```python
from build123d import *

# Parameters (mm, degrees)
F0_W     = 47.9163888
F0_H     = 16.881729
F1_DEPTH = 12.7
F2_R     = 8.382
F3_SIZE  = 8.382


# Not quite as in the source:
# - a feature names something its author has since deleted; it is built from what else it names


with BuildPart() as f1:
    # F0 (on Front) → F1 (new body, symmetric)
    with BuildSketch(Plane.XZ):
        Rectangle(F0_W, F0_H)
    extrude(amount=F1_DEPTH, both=True)

    # F2
    f2_edges = [f1.edges().sort_by_distance(p)[0] for p in [
        (0, -12.7, 8.440864),
        (0, -12.7, -8.440865),
        (-23.958194, -12.7, 0),
        (23.958194, -12.7, 0),
    ]]
    fillet(f2_edges, radius=F2_R)

    # F3
    f3_edges = [f1.edges().sort_by_distance(p)[0] for p in [
        (0, 12.7, 8.440864),
        (23.958194, 12.7, 0),
        (0, 12.7, -8.440865),
        (-23.958194, 12.7, 0),
    ]]
    chamfer(f3_edges, length=F3_SIZE)


solid = f1.part
```
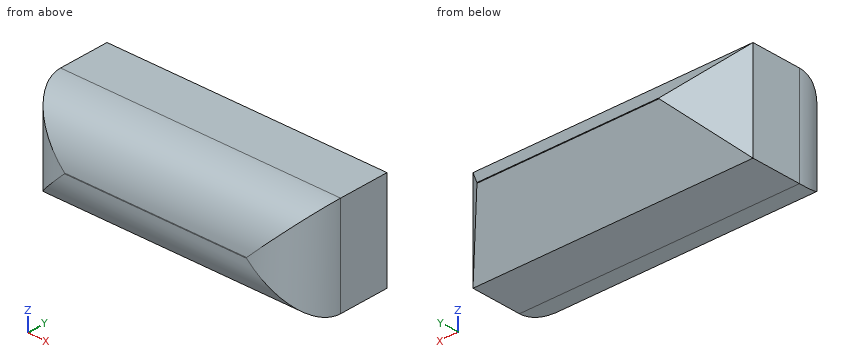
The listing builds one solid part. Answer for the finished solid, in the listing's coordinates (mm). Give positions to 0.01 mm unless a question says otherwise; leave off trailing zeros. Loops run counter-clockwise (first coordinate to the right, second up) from the corner with the lowest first, then second, coordinate; pieces in that order, holes last. Notation, with made-up numbers: (67.5, -16.5) - (108.5, -16.5) arc R15 ccw to (108.5, 10.5) - close; hole circle Ø1 at (-32, 31.25). An arc over 180 degrees is marked (long way). Return JSON: item names as keys, results as strings. Group by question number.
1. Find section B-B (z = 2.75). Write down the section's boundary in (x, y), then the cut area to 3 significant figures.
2. Find section C-C (y = -6.5). Write down the section's boundary in (x, z).
3. Straight lines are drawn through the part: line 1 (Z direction, x = -15.5, y = -6.5); line 2 (Y direction, x = 13, z = -2); line 3 (Y direction, x = -13.5, z = 1.25). For each, find the intervals that lie inside material, in ascending order. Write a range as [from, to].
4. Given pin 1 Ø3 at (x, z) = (15, -6.5) entering from -Y; pin 2 Ø2 at (x, y) = (16.5, 9) entering from +Z, each flat-ended and moving along its own axis, determine where each tip first touches the part or whether it passes through.
5. Find section A-A (x = 5.5). Write down the section's boundary in (y, z).
6. Find section D-D (y = 8.25). Write down the section's boundary in (x, z).
Verdict:
{
 "1": {"outline": "(-23.96, -4.32) arc R8.38 ccw to (-18.27, -12.26) - (18.27, -12.26) arc R8.38 ccw to (23.96, -4.32) - (23.96, 4.32) - (18.27, 10.01) - (-18.27, 10.01) - (-23.96, 4.32) - close", "area": "1,010 mm^2"},
 "2": {"outline": "(-23.67, -8.15) - (23.67, -8.15) - (23.67, 8.15) - (-23.67, 8.15) - close"},
 "3": {"line 1": "z = [-8.15, 8.15]", "line 2": "y = [-12.47, 10.76]", "line 3": "y = [-12.61, 11.51]"},
 "4": {"pin 1": "stops at y = -11.09", "pin 2": "stops at z = 4.76"},
 "5": {"outline": "(-12.7, -0.06) arc R8.38 ccw to (-4.32, -8.44) - (4.32, -8.44) - (12.7, -0.06) - (12.7, 0.06) - (4.32, 8.44) - (-4.32, 8.44) arc R8.38 ccw to (-12.7, 0.06) - close"},
 "6": {"outline": "(-20.03, -4.51) - (20.03, -4.51) - (20.03, 4.51) - (-20.03, 4.51) - close"}
}
